from build123d import *

# Parameters (mm, degrees)
SKETCH1_R                                           = 12
BOSS_EXTRUDE1_DEPTH                                 = 12
F_8_0MM_DOWEL_HOLE1_D                               = 8
CBORE_FOR_M2_HEX_SOCKET_HEAD_CAP_SCREW1_D           = 2.4
CBORE_FOR_M2_HEX_SOCKET_HEAD_CAP_SCREW1_CBORE_D     = 4.4
CBORE_FOR_M2_HEX_SOCKET_HEAD_CAP_SCREW1_CBORE_DEPTH = 5.5


with BuildPart() as part:
    # Sketch1 → Boss-Extrude1 (new body)
    with BuildSketch(Plane.XY):
        Circle(SKETCH1_R)
    extrude(amount=BOSS_EXTRUDE1_DEPTH)

    # Ø8.0mm Dowel Hole1 (through all)
    with Locations(Plane.XY.offset(12)):
        with Locations((0, 0)):
            Hole(F_8_0MM_DOWEL_HOLE1_D / 2)

    # CBORE for M2 Hex Socket Head Cap Screw1 (through all)
    with Locations(Plane(origin=(0, 0, 0), x_dir=(1, 0, 0), z_dir=(0, 0, -1))):
        with Locations((-5.656854249, -5.656854249), (0, -8), (5.656854249, -5.656854249), (8, 0), (5.656854249, 5.656854249), (0, 8), (-5.656854249, 5.656854249), (-8, 0)):
            CounterBoreHole(CBORE_FOR_M2_HEX_SOCKET_HEAD_CAP_SCREW1_D / 2, CBORE_FOR_M2_HEX_SOCKET_HEAD_CAP_SCREW1_CBORE_D / 2, CBORE_FOR_M2_HEX_SOCKET_HEAD_CAP_SCREW1_CBORE_DEPTH)


solid = part.part
The listing builds one solid part. Answer for the finished solid, in the listing's coordinates (mm). A direction names the side the tool comes from. Round coordinates to 2 decimals unless told otherwise and drop trailing zeros. Order: outer loops, then holes, each group sorted by start corner. A loop starts at its lowest first (then second) coordinate and runs counter-clockwise, first axis right, second up. Notation, with made-up numbers: (78.5, 29.5) -> (129.5, 29.5) arc R21 cw to (129.5, 39.5) -> close; hole circle Ø3 at (7.25, -24). An arc over 180 degrees is marked (long way). Write each question's results on one line, items separated by ' | '. Start each with the question number.
Q1. Find section C-C (y = -8.75). Determine the outline of the cut face in (x, z).
Q2. Which of the six approach directions +Z, -Z, +X, -X, +Y, -Y give full straight-line access (tool end or side, diameter ignored) to faces 1 (the flat face through (-7, 1, 5.5)), 2 (the cylindrical face through (6.856, 5.604, 8.796))?
Q3. The mould has two halves that part along Y. Classify faces 3 (the flat face through (-3, 3, 12)), 4 (the cylindrical face through (-4.46, 5.6, 8.8)): pulls with the +Y half, pulls with the -Y half, needs draft (parallel to the pull), parting line crosses it, or undercut.
Q4. Find section D-D (x = -5.5). Determine the outline of the cut face in (y, z), then the cut area to 3 significant figures.
Q5. Find section A-A (x = 0). Determine the outline of the cut face in (y, z), then the cut area to 3 significant figures.
Q6. Each of these flat-tipped pins is pushed along its axis until it touches: pin 1 (2 mm diameter, centred on y = -7, z = 5.5, fed in from +X); pin 2 (2 mm diameter, centred on x = 1, y = -8.5, fed in from -Z); pin 3 (4 mm diameter, centred on x = 3.5, z = 5, fed in from -Y); pin 4 (5.5 mm diameter, centred on x = -8, y = 0, fed in from -Z). Where does it stop, or does it pass through?
Q7. Straight lines are drawn through the part: probe 1 along Y at (x, z) = (0, 3.85); probe 2 along Y at (x, z) = (0, 10.25); probe 3 along X at (y, z) = (-5, 10.75). For each, find the intervals that lie inside material, in ascending order. Write a range as from..to.
Worked answers:
1) outline: (-8.21, 0) -> (-2.07, 0) -> (-2.07, 5.5) -> (-0.94, 5.5) -> (-0.94, 12) -> (-8.21, 12) -> close; (0.94, 5.5) -> (2.07, 5.5) -> (2.07, 0) -> (8.21, 0) -> (8.21, 12) -> (0.94, 12) -> close
2) face 1: -Z | face 2: +Z, -Z
3) face 3: needs draft | face 4: undercut
4) outline: (-10.67, 0) -> (-7.85, 0) -> (-7.85, 5.5) -> (-6.85, 5.5) -> (-6.85, 12) -> (-10.67, 12) -> close; (-4.47, 5.5) -> (-3.46, 5.5) -> (-3.46, 0) -> (3.46, 0) -> (3.46, 5.5) -> (4.47, 5.5) -> (4.47, 12) -> (-4.47, 12) -> close; (6.85, 5.5) -> (7.85, 5.5) -> (7.85, 0) -> (10.67, 0) -> (10.67, 12) -> (6.85, 12) -> close | area: 177 mm2
5) outline: (-12, 0) -> (-10.2, 0) -> (-10.2, 5.5) -> (-9.2, 5.5) -> (-9.2, 12) -> (-12, 12) -> close; (-6.8, 5.5) -> (-5.8, 5.5) -> (-5.8, 0) -> (-4, 0) -> (-4, 12) -> (-6.8, 12) -> close; (4, 0) -> (5.8, 0) -> (5.8, 5.5) -> (6.8, 5.5) -> (6.8, 12) -> (4, 12) -> close; (9.2, 5.5) -> (10.2, 5.5) -> (10.2, 0) -> (12, 0) -> (12, 12) -> (9.2, 12) -> close | area: 112 mm2
6) pin 1: stops at x = 10.39 | pin 2: stops at z = 5.5 | pin 3: stops at y = -11.91 | pin 4: stops at z = 0
7) probe 1: y = -12..-10.2, -5.8..-4, 4..5.8, 10.2..12 | probe 2: y = -12..-9.2, -6.8..-4, 4..6.8, 9.2..12 | probe 3: x = -10.91..-6.66, -4.65..4.65, 6.66..10.91
